Verification items for the finished model (mm, model axes). Coordinates: 2 decimals unless noted, no trailing zeros. Write each loop counter-clockwise with the first axis right and the second up, starting at its lowest first coordinate (ties: lowest second). Pieces come first, ordered by that corner, then holes. Notation, with made-up numbers: M 4,47 L 46,47 A10 cw 46,54 Z; hole C 40.25,86 d3. An arc over 180 degrees is marked long. One line per item, written item: value.
Solid Edge part; units mm, degrees
sketch "Sketch1" plane through (0, 0, 0) normal (0, 0, 1) x (1, 0, 0)
  line L0 (45, -40) -> (-45, -40)
  line L1 (-45, -40) -> (-45, 40)
  line L2 (-45, 40) -> (45, 40)
  line L3 (45, 40) -> (45, -40)
  line L4 (27.75, -14.5) -> (-27.75, -14.5)
  line L5 (-27.75, -14.5) -> (-27.75, 14.5)
  line L6 (-27.75, 14.5) -> (27.75, 14.5)
  line L7 (27.75, 14.5) -> (27.75, -14.5)
  dimension "D1" = 45
  dimension "D2" = 45
extrude "Protrusion1" add sketch "Sketch1" against normal blind 3
fillet "Round_1" radius 5 4 edges at (45, -40, -1.5) (45, 40, -1.5) (-45, 40, -1.5) (-45, -40, -1.5)
extrude "Cutout1" [suppressed]
sketch "Sketch2" plane through (0, 0, 0) normal (0, 0, 1) x (0, 1, 0)
  line L0 (-36, -7.25) -> (-23.5, -7.25)
  line L1 (-23.5, -7.25) -> (-23.5, -35)
  line L2 (-23.5, -35) -> (-36, -35)
  line L3 (-36, -35) -> (-36, -7.25)
  line L4 (36, -35) -> (23.5, -35)
  line L5 (23.5, -35) -> (23.5, -7.25)
  line L6 (23.5, -7.25) -> (36, -7.25)
  line L7 (36, -7.25) -> (36, -35)
  line L8 (23.5, 35) -> (36, 35)
  line L9 (36, 35) -> (36, -3.25)
  line L10 (36, -3.25) -> (23.5, -3.25)
  line L11 (23.5, -3.25) -> (23.5, 35)
  line L12 (-36, 35) -> (-23.5, 35)
  line L13 (-23.5, 35) -> (-23.5, -3.25)
  line L14 (-23.5, -3.25) -> (-36, -3.25)
  line L15 (-36, -3.25) -> (-36, 35)
  line L16 (17.5, 31.75) -> (-17.5, 31.75)
  line L17 (-17.5, 31.75) -> (-17.5, 41)
  line L18 (-17.5, 41) -> (17.5, 41)
  line L19 (17.5, 41) -> (17.5, 31.75)
  line L20 (17.5, -41) -> (-17.5, -41)
  line L21 (-17.5, -41) -> (-17.5, -33.25)
  line L22 (-17.5, -33.25) -> (17.5, -33.25)
  line L23 (17.5, -33.25) -> (17.5, -41)
  dimension "D1" = 36
  dimension "D2" = 36
extrude "Cutout2" cut sketch "Sketch2" against normal through all
fillet "Round_2" radius 2 28 edges at (-35, -23.5, -1.5) (3.25, -23.5, -1.5) (3.25, -36, -1.5) (-35, -36, -1.5) (7.25, -36, -1.5) (7.25, -23.5, -1.5) (35, -23.5, -1.5) (35, -36, -1.5) (35, 23.5, -1.5) (35, 36, -1.5) (7.25, 36, -1.5) (7.25, 23.5, -1.5) (3.25, 36, -1.5) (3.25, 23.5, -1.5) (-35, 36, -1.5) (-35, 23.5, -1.5) (-27.75, 14.5, -1.5) (-27.75, -14.5, -1.5) (27.75, 14.5, -1.5) (27.75, -14.5, -1.5) (-41, 17.5, -1.5) (-31.75, 17.5, -1.5) (-31.75, -17.5, -1.5) (-41, -17.5, -1.5) (33.25, -17.5, -1.5) (41, -17.5, -1.5) (41, 17.5, -1.5) (33.25, 17.5, -1.5)
hole "Hole_1" at (-18.75, -17.3, -3) direction (0, 0, 1) diameter 2.5 end up to next countersink diameter 5 countersink angle 90
hole "Hole1" at (3.25, -17.3, -3) direction (0, 0, 1) diameter 2.5 end up to next countersink diameter 5 countersink angle 90
hole "Hole2" at (25.25, -17.3, -3) direction (0, 0, 1) diameter 2.5 end up to next countersink diameter 5 countersink angle 90
hole "Hole3" at (25.25, 17.3, -3) direction (0, 0, 1) diameter 2.5 end up to next countersink diameter 5 countersink angle 90
hole "Hole4" at (3.25, 17.3, -3) direction (0, 0, 1) diameter 2.5 end up to next countersink diameter 5 countersink angle 90
hole "Hole5" at (-18.75, 17.3, -3) direction (0, 0, 1) diameter 2.5 end up to next countersink diameter 5 countersink angle 90
properties material "ABS Plastic, medium impact"
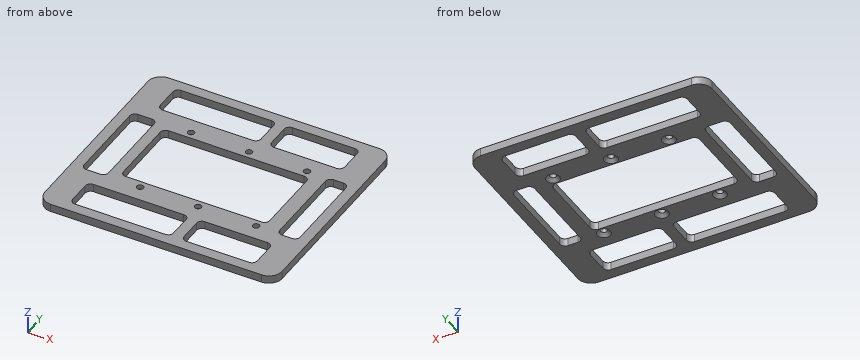
Item 1: Cross-section at A-A, the plane y = -30. Enter the section's corners in (x, z), and give its area (3 significant figures).
The answers:
outline: M -45,-3 L -35,-3 L -35,0 L -45,0 Z; M 3.25,-3 L 7.25,-3 L 7.25,0 L 3.25,0 Z; M 35,-3 L 45,-3 L 45,0 L 35,0 Z
area: 72.0 mm²
Item 2: Scan lines: line 1 (Y direction, x = -14, z = -2.3); line 2 (X direction, y = -11, z = -1.45); line 3 (X direction, y = -29.5, z = -1.2). Record each from-to range of solid material in increasing order.
The answers:
line 1: y = -40 to -36, -23.5 to -14.5, 14.5 to 23.5, 36 to 40
line 2: x = -45 to -41, -31.75 to -27.75, 27.75 to 33.25, 41 to 45
line 3: x = -45 to -35, 3.25 to 7.25, 35 to 45
Item 3: Cross-section at C-C, the plane x = 30. Enter the section's corners in (y, z).
The answers:
outline: M -40,-3 L -36,-3 L -36,0 L -40,0 Z; M -23.5,-3 L 23.5,-3 L 23.5,0 L -23.5,0 Z; M 36,-3 L 40,-3 L 40,0 L 36,0 Z
Item 4: Cross-section at D-D, the plane z = -1.1. Give the number of separate pieces and of enclosed holes in the cut face, and give its area (3 significant figures).
The answers:
separate pieces: 1
enclosed holes: 13
area: 3,320 mm²
Item 5: Cross-section at B-B, the plane x = -24.5. Enter the section's corners in (y, z), and give its area (3 significant figures).
The answers:
outline: M -40,-3 L -36,-3 L -36,0 L -40,0 Z; M -23.5,-3 L -14.5,-3 L -14.5,0 L -23.5,0 Z; M 14.5,-3 L 23.5,-3 L 23.5,0 L 14.5,0 Z; M 36,-3 L 40,-3 L 40,0 L 36,0 Z
area: 78.0 mm²
Item 6: Go/stop test with flat-tipped pins: P1, Ø3, axis at x = 25.25, y = 17.3, coming from the -Z side; P2, Ø3, axis at x = 25.25, y = -17.3, coming from the +Z side; P3, Ø2, axis at x = -18.75, y = -17.3, coming from the +Z side. Record where each tip stops, or that it passes through.
The answers:
P1: stops at z = -2
P2: stops at z = 0
P3: passes through
